Check sheet for the modelled part. Datum: model origin and axes. Units: mm. Face numbers are marked on the shaded views. A direction names the side the tool comes from. Coordinates: 2 decimals unless noted, no trailing zeros. Loops run counter-clockwise (first coordinate to the right, second up) from the corner with the lowest first, then second, coordinate; pieces in that order, holes last. Notation, with made-up numbers: M -24.75,22 L -17.75,22 A30 cw -17.75,59 Z; hole C 64.5,32.25 d5. An arc over 180 degrees is marked long. Answer as CSV lines item,"result". Start each with the question number.
Autodesk Inventor part; units mm, degrees
ref_plane "Work Plane1" through (1.525, 0, 0) normal (0, 0, 1) x (1, 0, 0)
ref_plane "YZ Plane" through (0, 0, 0) normal (1, 0, 0) x (0, 1, 0)
ref_plane "XZ Plane" through (0, 0, 0) normal (0, 1, 0) x (-1, 0, 0)
sketch "Sketch1" plane through (0, 0, 0) normal (0, 0, 1) x (1, 0, 0)
  line L0 (0, 6.4294) -> (0, 4.7625)
  line L1 (31.75, 4.7625) -> (57.15, 4.7625)
  line L2 (57.15, 4.7625) -> (57.15, 0)
  line L3 (57.15, 0) -> (-0.6351, 0)
  line L4 (-12.1921, 0) -> (68.707, 0)
  line L5 (-0.6351, 0) -> (-0.6351, 6.4294)
  line L6 (-0.6351, 6.4294) -> (0, 6.4294)
  line L7 (31.75, 4.7625) -> (30.1624, 4.7625)
  line L8 (30.1624, 4.7625) -> (0, 4.7625)
  line L9 (0, -1.2859) -> (0, 7.7152)
  dimension "d0" = 57.15
  dimension "d1" = 25.4
  dimension "d2" = 9.525
  dimension "d9" = 0.6351
  dimension "d10" = 12.8588
  dimension "d13" = 1.5876
  dimension "d14" = 9.525
revolve "Body" add sketch "Sketch1" angle 360 about axis through (57.15, 0, 0) along (-1, 0, 0)
sketch "Sketch2" plane through (-0.6351, 0, 0) normal (-1, 0, 0) x (0, 0, 1)
  line L0 (0, 8.2489) -> (7.1437, 4.1244)
  line L1 (7.1437, 4.1244) -> (7.1437, -4.1244)
  line L2 (7.1437, -4.1244) -> (0, -8.2489)
  line L3 (0, -8.2489) -> (-7.1437, -4.1244)
  line L4 (-7.1437, -4.1244) -> (-7.1437, 4.1244)
  line L5 (-7.1437, 4.1244) -> (0, 8.2489)
  point P0 (0, 0)
  point P1 (0, 0)
  dimension "d11" = 14.2875
extrude "Head" add sketch "Sketch2" along normal blind 5.3181
sketch "Sketch4" plane through (0, 0, 0) normal (0, 0, 1) x (1, 0, 0)
  line L0 (-5.9532, 7.1437) -> (-5.9532, 8.2489)
  line L1 (-5.9532, 8.2489) -> (-5.3152, 8.2489)
  line L2 (-5.3152, 8.2489) -> (-5.9532, 7.1437)
  line L3 (-7.0169, 0) -> (0.4285, 0)
  line L4 (-0.6351, 8.2489) -> (-5.9532, 8.2489)
  line L5 (-5.9532, 4.1244) -> (-5.9532, 8.2489)
  dimension "d5" = 30
  dimension "d19" = 14.2875
revolve "Chamfer1" cut sketch "Sketch4" angle 360 about axis through (-10, 0, 0) along (1, 0, 0)
thread "Thread"
chamfer "Chamfer2" distance 0.8593 distance2 1.5876 1 edges at (57.15, -4.7625, 0) measured on face at (57.15, 0.9018, -1.6622)
ref_plane "Work Plane1" through (1.525, 0, 0) normal (0, 0, 1) x (1, 0, 0)
fillet "Fillet2" radius 0.635 1 edges at (0, -4.7625, 0)
equation "\"d0\" = NLG"
equation "\"d1\" = GEL"
equation "\"d2\" = GD"
equation "\"d10\" = SD2"
equation "\"d14\" = BDM"
equation "\"d11\" = SW"
equation "\"d3\" = KOH - SD"
equation "\"d5\" = ANG1"
equation "\"d19\" = SW0"
equation "\"d63\" = R"
equation "\"d15\" = GEL"
equation "\"d6\" = -0.5 * SPD + 0.5 * GD"
equation "\"NLG\" = 57.15"
equation "\"GD\" = NND"
equation "\"BDM\" = 9.525"
equation "\"KOH\" = 5.95312"
equation "\"GEL\" = 25.4"
equation "\"SW\" = 14.2875"
equation "\"SW0\" = SW"
equation "\"SPD\" = 7.80644"
equation "\"SD2\" = 12.85875"
equation "\"SD\" = 0.635"
equation "\"ANG1\" = 30deg"
equation "\"GAL\" = 1.5875"
equation "\"GUL\" = 1.5875"
equation "\"R\" = 0.635"
equation "\"THREADDIA\" = 9.525"
equation "\"TOA\" = 30deg"
equation "\"RR\" = 0.508"
equation "\"NND\" = 9.525"
equation "\"E0\" = 1.155 * SW"
equation "\"SLG\" = 0"
equation "\"GD1\" = 7.80644"
properties part number "ANSI B18.2.1 - 3/8-16 UNC - 2.25, HCSI" material "Steel, Mild"
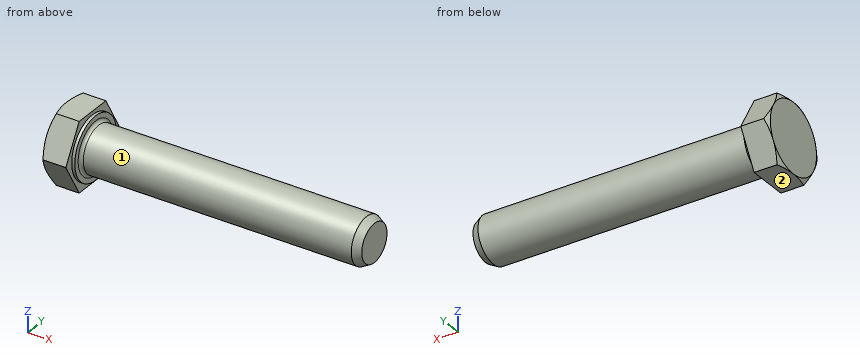
Item 1: Sectioned sample at A-A, the plane x = 39. Record the boundary of the cut face in (y, z) (1 decimal), and give its area (3 significant figures).
Item 2: Set-up check for the marked faces 1 and 2: record each of +Z, -Z, +X, -X, +Y, -Y from which the full face is reachable in a straight line by a thin tool's end or side.
Item 3: Material ranges on line 1 (X direction, y = 2.75, z = 5.5); line 2 (Z direction, x = 42, y = 0); line 3 (Z direction, x = -2, y = -6), recorded low to high. Write a range as from..to.
Item 4: Go/stop test with flat-tipped pins: pin 1 (3 mm diameter, centred on x = 39, z = -3.5, fed in from +Y); pin 2 (2 mm diameter, centred on x = 7, z = -5, fed in from +Y); pin 3 (1 mm diameter, centred on x = 3, z = 0, fed in from -Y). Record where each tip stops, or that it passes through.
Reply:
1,outline,"C 0,0 d9.5"
1,area,"71.3 mm²"
2,face 1,"+X"
2,face 2,"-Z, +X, -X, +Y, -Y"
3,line 1,"-5.95..0"
3,line 2,"-4.76..4.76"
3,line 3,"-3.9..3.9"
4,pin 1,"y = 4.32"
4,pin 2,"y = 2.58"
4,pin 3,"y = -4.76"
